For this review, take the finished solid that the model builds, in its own axes (mm). Face numbers are marked on the shaded views. A direction names the side the tool comes from. Coordinates: 2 decimals unless noted, no trailing zeros. Order: outer loops, then holes, each group sorted by start corner. A loop starts at its lowest first (then second) coordinate and runs counter-clockwise, first axis right, second up. Notation, with made-up numbers: (-5.5, 49) -> (17.5, 49) arc R24 ccw to (17.5, 70) -> close; hole circle Ø2 at (-14, -10.75). An arc over 180 degrees is marked (long way). Answer as a JSON object with one key per item and string values. Group by question number.
1) Draft analysis for pull direction Z (two halves, no side actions). For the marked faces 1, 2, 3 and 4, state which applies: +Z half, -Z half, draft (parallel to the pull), parting line (faces both ways), or undercut.
2) For pin 1 (12 mm diameter, centred on x = 13, z = 15.5, fed in from +Y); pin 2 (7 mm diameter, centred on y = -4, z = 12, fed in from +X); pin 3 (1 mm diameter, centred on x = -28, z = 42.5, fed in from -Y), all flat-tipped, find the tip position at first contact; note any pin that passes through.
3) Add section A-A, the plane y = 14.5. Write out the cut boundary in (x, z), then the cut area to 3 significant figures.
4) Add section C-C, the plane x = 7.5. Write out the cut boundary in (y, z).
5) Add section B-B, the plane x = 64. Write out the cut boundary in (y, z).
6) Wall thickness on L1, parallel to X at y = 17.5, z = 48.75; L2, parallel to Z at x = 36, y = 14.5; L3, parallel to Z at x = 62, y = 4.5: over which ranges is each line inside the solid? List them lowest first.
7) Machinability: for the marked faces 5, 6 and 7, which of the approach directions +Z, -Z, +X, -X, +Y, -Y give a long, thin tool a straight path to every point of the face, cutting with its end or side? Answer none if there is none.
from build123d import *

# Parameters (mm, degrees)
F0_R      = 7.75
F1_DEPTH  = 65
F2_R      = 6
F3_DEPTH  = 25
F4_W      = 15
F4_H      = 6
F5_DEPTH  = 25
F6_R      = 1.5
F7_DEPTH  = 25
F8_R      = 3.75
F8_R_2    = 1.45
F8_R_3    = 5.5
F9_DEPTH  = 7
F10_R     = 1.5
F11_DEPTH = 5
F2_W      = 53
F2_H      = 19
F2_W_2    = 19
F2_H_2    = 17
F12_DEPTH = 19.47049
F13_DEPTH = 17


with BuildPart() as f1:
    # F0 (on Top) → F1 (new body)
    with BuildSketch(Plane.XY):
        with BuildLine():
            Line((25, -7.470489), (32.163705, -9.589339))
            ThreePointArc((32.163705, -9.589339), (33.567065, -9.896802), (35, -10))
            ThreePointArc((35, -10), (42.071068, -7.071068), (45, 0))
            Line((45, 0), (45, 12))
            Line((45, 12), (0, 12))
            Line((0, 12), (-45, 12))
            Line((-45, 12), (-45, 0))
            ThreePointArc((-45, 0), (-40.984858, -8.011334), (-32.163705, -9.589339))
            Line((-32.163705, -9.589339), (-25, -7.470489))
            Line((-25, -7.470489), (-25, 0))
            Line((-25, 0), (-25, 1.5))
            ThreePointArc((-25, 1.5), (-23.535534, 5.035534), (-20, 6.5))
            Line((-20, 6.5), (20, 6.5))
            ThreePointArc((20, 6.5), (23.535534, 5.035534), (25, 1.5))
            Line((25, 1.5), (25, 0))
            Line((25, 0), (25, -7.470489))
        make_face()
        with Locations((-35, 0)):
            Circle(F0_R, mode=Mode.SUBTRACT)
        with Locations((35, 0)):
            Circle(F0_R, mode=Mode.SUBTRACT)
    extrude(amount=F1_DEPTH)

    # F2 (on face) → F3 (cut)
    with BuildSketch(Plane(origin=(0, 12, 0), x_dir=(-1, 0, 0), z_dir=(0, 1, 0))):
        with BuildLine():
            Line((-5.5, 65), (-5.5, 60))
            ThreePointArc((-5.5, 60), (0, 51.602084), (5.5, 60))
            Line((5.5, 60), (5.5, 65))
            Line((5.5, 65), (-5.5, 65))
        make_face()
        with Locations((0, 32.5)):
            Circle(F2_R)
        with BuildLine():
            Line((-5.5, 5), (-5.5, 0))
            Line((-5.5, 0), (5.5, 0))
            Line((5.5, 0), (5.5, 5))
            ThreePointArc((5.5, 5), (0, 13.397916), (-5.5, 5))
        make_face()
    extrude(amount=-F3_DEPTH, mode=Mode.SUBTRACT)

    # F4 (on face) → F5 (join)
    with BuildSketch(Plane.YZ.offset(45)):
        with Locations((4.5, 29.5)):
            Rectangle(F4_W, F4_H)
        with Locations((4.5, 3)):
            Rectangle(F4_W, F4_H)
    extrude(amount=F5_DEPTH)

    # F6 (on face) → F7 (cut)
    with BuildSketch(Plane(origin=(0, 0, 26.5), x_dir=(1, 0, 0), z_dir=(0, 0, -1))):
        with Locations((64, -4.5)):
            Circle(F6_R)
    extrude(amount=-F7_DEPTH, mode=Mode.SUBTRACT)

    # F8 (on face) → F9 (join)
    with BuildSketch(Plane(origin=(0, 12, 0), x_dir=(-1, 0, 0), z_dir=(0, 1, 0))):
        with Locations((31, 32.5)):
            Circle(F8_R)
        with Locations((31, 32.5)):
            Circle(F8_R_2, mode=Mode.SUBTRACT)
        with BuildLine():
            ThreePointArc((-35.999405, 56.75), (-30.343356, 43.092935), (-44, 48.75))
            Line((-44, 48.75), (-44, 13.75))
            ThreePointArc((-44, 13.75), (-30.343146, 19.406854), (-36, 5.75))
            Line((-36, 5.75), (-38.5, 5.75))
            ThreePointArc((-38.5, 5.75), (-39.914214, 5.164214), (-40.5, 3.75))
            Line((-40.5, 3.75), (-40.5, 0))
            Line((-40.5, 0), (-25.25, 0))
            Line((-25.25, 0), (-25.25, 65))
            Line((-25.25, 65), (-40.5, 65))
            Line((-40.5, 65), (-40.5, 58.750074))
            ThreePointArc((-40.5, 58.750074), (-39.914235, 57.335882), (-38.50006, 56.750074))
            Line((-38.50006, 56.750074), (-35.999405, 56.75))
        make_face()
        Polygon((-44, 65), (-45, 65), (-45, 32.5), (-45, 26.5), (-45, 6), (-45, 0), (-44, 0), (-44, 13.75), (-44, 48.75), align=None)
        with Locations((-36, 13.75)):
            Circle(F8_R_3)
        with BuildLine():
            ThreePointArc((-30.5, 48.75), (-36, 54.25), (-41.5, 48.75))
            ThreePointArc((-41.5, 48.75), (-36, 43.25), (-30.5, 48.75))
        make_face()
    extrude(amount=F9_DEPTH)

    # F10 (on face) → F11 (cut)
    with BuildSketch(Plane(origin=(-45, 0, 0), x_dir=(0, -1, 0), z_dir=(-1, 0, 0))):
        with Locations((-6, 26.5)):
            Circle(F10_R)
        with Locations((-6, 38.5)):
            Circle(F10_R)
    extrude(amount=-F11_DEPTH, mode=Mode.SUBTRACT)

    # F2 (on face) → F12 (join)
    with BuildSketch(Plane(origin=(0, 12, 0), x_dir=(-1, 0, 0), z_dir=(0, 1, 0))):
        with Locations((0, 32.5)):
            Rectangle(F2_W, F2_H)
        with Locations((0, 32.5)):
            Rectangle(F2_W_2, F2_H_2, mode=Mode.SUBTRACT)
        with Locations((0, 32.5)):
            Rectangle(F2_W_2, F2_H_2)
        with Locations((0, 32.5)):
            Circle(F2_R, mode=Mode.SUBTRACT)
    extrude(amount=-F12_DEPTH)

    # F2 (on face) → F13 (cut)
    with BuildSketch(Plane(origin=(0, 12, 0), x_dir=(-1, 0, 0), z_dir=(0, 1, 0))):
        with Locations((0, 32.5)):
            Rectangle(F2_W_2, F2_H_2)
        with Locations((0, 32.5)):
            Circle(F2_R, mode=Mode.SUBTRACT)
    extrude(amount=-F13_DEPTH, mode=Mode.SUBTRACT)


solid = f1.part
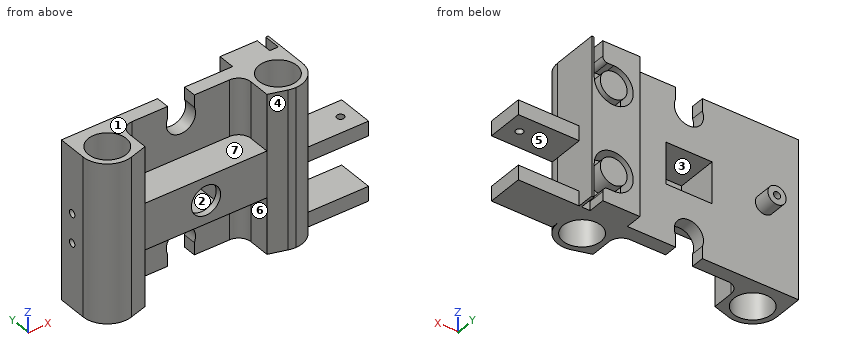
Output values:
{
 "1": {"face 1": "+Z half", "face 2": "undercut", "face 3": "undercut", "face 4": "draft"},
 "2": {"pin 1": "stops at y = 12", "pin 2": "stops at x = 44.99", "pin 3": "stops at y = -8.51"},
 "3": {"outline": "circle Ø7.5 at (-31, 32.5); (25.25, 0) -> (40.5, 0) -> (40.5, 3.75) arc R2 ccw to (38.5, 5.75) -> (36, 5.75) arc R8 cw (long way) to (44, 13.75) -> (44, 0) -> (45, 0) -> (45, 65) -> (44, 65) -> (44, 48.75) arc R8 cw (long way) to (36, 56.75) -> (38.5, 56.75) arc R2 ccw to (40.5, 58.75) -> (40.5, 65) -> (25.25, 65) -> close; circle Ø11 at (36, 13.75); circle Ø11 at (36, 48.75); hole circle Ø2.9 at (-31, 32.5)", "area": "1,030 mm²"},
 "4": {"outline": "(-7.47, 23) -> (6.5, 23) -> (6.5, 0) -> (12, 0) -> (12, 24) -> (-5, 24) -> (-5, 41) -> (12, 41) -> (12, 65) -> (6.5, 65) -> (6.5, 42) -> (-7.47, 42) -> close"},
 "5": {"outline": "(-3, 0) -> (12, 0) -> (12, 6) -> (-3, 6) -> close; (-3, 26.5) -> (3, 26.5) -> (3, 32.5) -> (-3, 32.5) -> close; (6, 26.5) -> (12, 26.5) -> (12, 32.5) -> (6, 32.5) -> close"},
 "6": {"L1": "x = 25.25 to 28, 30.5 to 41.5, 44 to 45", "L2": "z = 0 to 5.75, 8.25 to 19.25, 21.75 to 40.75, 43.25 to 54.25, 56.75 to 65", "L3": "z = 0 to 6, 26.5 to 32.5"},
 "7": {"face 5": "+X, +Y, -Y", "face 6": "-Z, -Y", "face 7": "+Z, -Y"}
}
